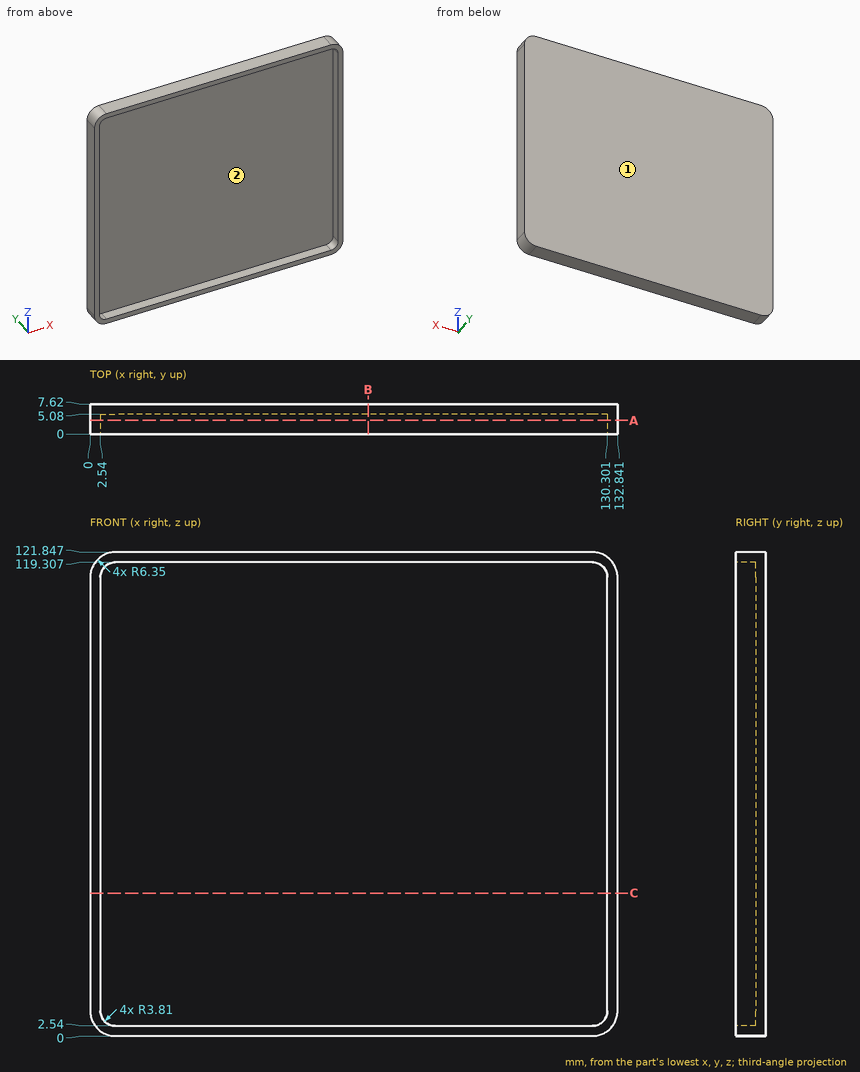
Study the drawing (mm; zero at the part's minimum x, y, z) and answer. Round coordinates to 2 decimals unless told otherwise and drop trailing zeros. Write each loop counter-clockwise with the first axis right and the second up, starting at its lowest first coordinate (ties: lowest second). Pieces come first, ordered by that corner, then holes. Notation, with made-up numbers: (-5.5, 2) - (38.5, 2) arc R31 ccw to (38.5, 30) - close; hole circle Ø2 at (15, 21.25). An arc over 180 degrees is marked (long way). Use a Markdown table: item, result. Add a question column.
1. Consider line 1 (Z direction, x = 72, y = 4); line 2 (X direction, y = 1.25, z = 40); line 3 (Y direction, x = 25.5, z = 20). Determine where each line is inside the solid, lowest interval first.
2. For a pull along Z with two mould halves and no side action, classify the marked faces 1 and 2 as +Z half, -Z half, draft (parallel to the pull), parting line (faces both ways), or undercut.
3. The part is cut by section B-B (x = 70). Write down the section's boundary in (y, z), and give its area (3 significant figures).
4. The part is cut by section C-C (z = 36). Write down the section's boundary in (x, y).
5. The part is cut by section A-A (y = 3.5). Write down the section's boundary in (x, z).
6. A flat-ended cylindrical pin translates along its axis: P1, Ø5, axis at x = 52, z = 16.5, coming from the -Y side. Find the tip coordinate at first contact, or state that the pin passes through.
Reported:
| question | item | result |
|---|---|---|
| 1 | line 1 | 0 to 2.54, 119.31 to 121.85 |
| 1 | line 2 | 0 to 2.54, 130.3 to 132.84 |
| 1 | line 3 | 5.08 to 7.62 |
| 2 | face 1 | draft |
| 2 | face 2 | undercut |
| 3 | outline | (0, 0) - (7.62, 0) - (7.62, 121.85) - (0, 121.85) - (0, 119.31) - (5.08, 119.31) - (5.08, 2.54) - (0, 2.54) - close |
| 3 | area | 335 mm^2 |
| 4 | outline | (0, 0) - (2.54, 0) - (2.54, 5.08) - (130.3, 5.08) - (130.3, 0) - (132.84, 0) - (132.84, 7.62) - (0, 7.62) - close |
| 5 | outline | (0, 6.35) arc R6.35 ccw to (6.35, 0) - (126.49, 0) arc R6.35 ccw to (132.84, 6.35) - (132.84, 115.5) arc R6.35 ccw to (126.49, 121.85) - (6.35, 121.85) arc R6.35 ccw to (0, 115.5) - close; hole (2.54, 6.35) arc R3.81 ccw to (6.35, 2.54) - (126.49, 2.54) arc R3.81 ccw to (130.3, 6.35) - (130.3, 115.5) arc R3.81 ccw to (126.49, 119.31) - (6.35, 119.31) arc R3.81 ccw to (2.54, 115.5) - close |
| 6 | P1 | y = 5.08 |
